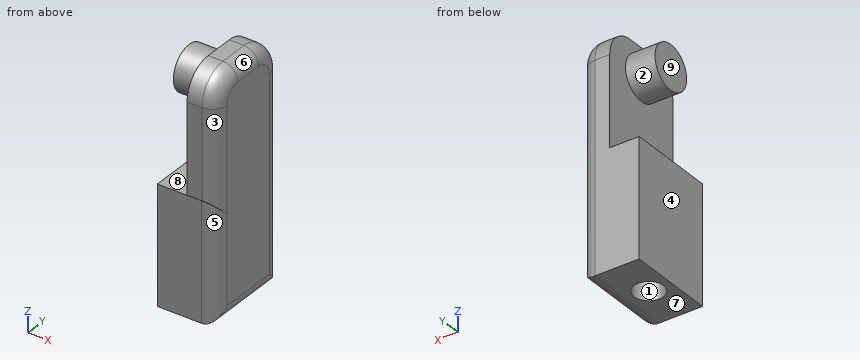
```python
from build123d import *

# Parameters (mm, degrees)
SKETCH1_W           = 40.43076923
SKETCH1_H           = 30
BOSS_EXTRUDE1_DEPTH = 10
SKETCH2_R           = 7.5
BOSS_EXTRUDE2_DEPTH = 20
FILLET1_R           = 10
CUT_EXTRUDE1_START  = -10
SKETCH3_R           = 7.5
CUT_EXTRUDE1_DEPTH  = 10
SKETCH4_W           = 20
SKETCH4_H           = 30.102362665
BOSS_EXTRUDE3_DEPTH = 40
FILLET2_R           = 5
SKETCH5_R           = 5
CUT_EXTRUDE2_DEPTH  = 10


with BuildPart() as part:
    # Sketch1 → Boss-Extrude1 (new body)
    with BuildSketch(Plane(origin=(0, 0, 0), x_dir=(0, 0, -1), z_dir=(1, 0, 0))):
        Rectangle(SKETCH1_W, SKETCH1_H)
    extrude(amount=BOSS_EXTRUDE1_DEPTH)

    # Sketch2 → Boss-Extrude2 (add)
    with BuildSketch(Plane.ZY):
        with Locations(Location((10.107692308, 0, 0), (0, 0, 180))):
            Circle(SKETCH2_R)
    extrude(amount=BOSS_EXTRUDE2_DEPTH)

    # Fillet1
    fillet1_edges = [part.edges().sort_by_distance(p)[0] for p in [
        (5, -15, 20.215384615),
        (5, 15, 20.215384615),
    ]]
    fillet(fillet1_edges, radius=FILLET1_R)

    # Sketch3 → Cut-Extrude1 (cut)
    with BuildSketch(Plane.ZY.offset(20).offset(CUT_EXTRUDE1_START)):
        with Locations(Location((10.107692308, 0, 0), (0, 0, 180))):
            Circle(SKETCH3_R)
    extrude(amount=CUT_EXTRUDE1_DEPTH, mode=Mode.SUBTRACT)

    # Sketch4 → Boss-Extrude3 (add)
    with BuildSketch(Plane(origin=(0, 0, -20.215384615), x_dir=(-1, 0, 0), z_dir=(0, 0, -1))):
        with Locations((0, -0.051181332)):
            Rectangle(SKETCH4_W, SKETCH4_H)
    extrude(amount=BOSS_EXTRUDE3_DEPTH)

    # Fillet2
    fillet2_edges = [part.edges().sort_by_distance(p)[0] for p in [
        (10, -15, -5),
        (10, 0, 20.215384615),
        (10, 12.071067812, 17.286452427),
        (10, -12.071067812, 17.286452427),
        (10, -15.051181332, -20.215384615),
        (10, -15.102362665, -40.215384615),
        (10, -0.051181332, -60.215384615),
        (10, 15, -25),
    ]]
    fillet(fillet2_edges, radius=FILLET2_R)

    # Sketch5 → Cut-Extrude2 (cut)
    with BuildSketch(Plane(origin=(0, 0, -60.215384615), x_dir=(-1, 0, 0), z_dir=(0, 0, -1))):
        with Locations((2.5, -0.051181332)):
            Circle(SKETCH5_R)
    extrude(amount=-CUT_EXTRUDE2_DEPTH, mode=Mode.SUBTRACT)


solid = part.part
```
Could you check a few things on this model? Use its own coordinates, in mm. Face numbers are marked on the shaded views. A direction names the side the tool comes from. Give positions to 0.01 mm unless a question says otherwise; leave off trailing zeros. Loops run counter-clockwise (first coordinate to the right, second up) from the corner with the lowest first, then second, coordinate; pieces in that order, holes last. Notation, with made-up numbers: (-27.5, 43) - (-18.5, 43) arc R32 cw to (-18.5, 70) - close; hole circle Ø8 at (47.5, -10.75). An arc over 180 degrees is marked (long way). Answer in a Markdown table with one row per item. Add a question column.
Q1. We'd pull the mould along Z, two halves only. Please class the marked faces 6, 7, 8 and 9: +Z half, -Z half, draft (parallel to the pull), parting line (faces both ways), or undercut.
Q2. For pin 1 (5 mm diameter, centred on y = 12, z = -16, fed in from -X); pin 2 (3 mm diameter, centred on x = 3.5, y = -7, fed in from +Z); pin 3 (4 mm diameter, centred on x = 1.5, z = -4.5, fed in from -Y), each with a flat end and sliding along its axis, tell me the tip position at first contact or that it passes through.
Q3. If we section it at C-C (x = 3.75): List the corners of the cut face in (y, z) for me, plus the area to 3 significant figures.
Q4. Please list where these lines run through material, in increasing order: L1, parallel to Y at x = -2.5, z = -56; L2, parallel to X at y = 6.5, z = -5.5; L3, parallel to Z at x = -8.75, y = -9. Write a range as from..to.
Q5. Which directions (+Z, -Z, +X, -X, +Y, -Y) give clear straight access to the entire face, cutting with the end or side of a thin tool? Please do the marked faces 1, 2, 3, 4 and 5.
Q6. If we section it at B-B (z = -30.5): List the corners of the cut face in (x, y) for me.
Q7. If we section it at A-A (x = -2.5): List the corners of the cut face in (y, z) for me.
Q8. If we section it at D-D (y = 3): List the corners of the cut face in (x, z) for me.
The answers:
| question | item | result |
|---|---|---|
| 1 | face 6 | +Z half |
| 1 | face 7 | -Z half |
| 1 | face 8 | undercut |
| 1 | face 9 | draft |
| 2 | pin 1 | stops at x = 0 |
| 2 | pin 2 | stops at z = 20.2 |
| 2 | pin 3 | stops at y = -15 |
| 3 | outline | (-15.1, -60.22) - (15, -60.22) - (15, 10.22) arc R10 ccw to (5, 20.22) - (-5, 20.22) arc R10 ccw to (-15, 10.22) - (-15, -20.22) - (-15.1, -20.22) - close |
| 3 | area | 2,370 mm^2 |
| 4 | L1 | y = -15.1..-5.05, 4.95..15 |
| 4 | L2 | x = 0..10 |
| 4 | L3 | z = -60.22..-20.22 |
| 5 | face 1 | -Z |
| 5 | face 2 | -X |
| 5 | face 3 | +Z, +X, -Y |
| 5 | face 4 | +Z, -Z, -X, +Y, -Y |
| 5 | face 5 | +Z, -Z, +X, -Y |
| 6 | outline | (-10, -15.1) - (5, -15.1) arc R5 ccw to (10, -10.1) - (10, 10) arc R5 ccw to (5, 15) - (-10, 15) - close |
| 7 | outline | (-15.1, -60.22) - (-5.05, -60.22) - (-5.05, -50.22) - (4.95, -50.22) - (4.95, -60.22) - (15, -60.22) - (15, -20.22) - (-15.1, -20.22) - close; circle Ø15 at (0, 10.11) |
| 8 | outline | (-10, -60.22) - (-6.46, -60.22) - (-6.46, -50.22) - (1.46, -50.22) - (1.46, -60.22) - (5, -60.22) arc R5 ccw to (10, -55.22) - (10, 15.22) arc R5 ccw to (5, 20.22) - (0, 20.22) - (0, 16.98) - (-10, 16.98) - (-10, 3.23) - (0, 3.23) - (0, -20.22) - (-10, -20.22) - close |
